Geometry check sheet. Reference: the model listing, model coordinates, mm. A direction names the side the tool comes from. Give positions to 0.01 mm unless a question says otherwise; leave off trailing zeros. Loops run counter-clockwise (first coordinate to the right, second up) from the corner with the lowest first, then second, coordinate; pieces in that order, holes last. Notation, with made-up numbers: (-25.75, -23) -> (21.25, -23) arc R20 ccw to (21.25, -14) -> close; hole circle Ø6 at (28, -33). An arc over 180 degrees is marked (long way). Answer as a JSON object with one key per item and string values.
Autodesk Inventor part; units mm, degrees
ref_plane "YZ Plane" through (0, 0, 0) normal (1, 0, 0) x (0, 1, 0)
ref_plane "XZ Plane" through (0, 0, 0) normal (0, 1, 0) x (-1, 0, 0)
ref_plane "XY Plane" through (0, 0, 0) normal (0, 0, 1) x (1, 0, 0)
sketch "Sketch1" plane through (0, 0, 0) normal (0, 0, 1) x (1, 0, 0)
  circle A0 centre (0, 0) radius 10.16
  circle A1 centre (0, 0) radius 8.7376
  dimension "d0" = 20.32
  dimension "d6" = 17.4752
extrude "Extrusion1" add sketch "Sketch1" along normal blind 12.7 contours A0 | A1
sketch "Sketch2" plane through (0, 0, 12.7) normal (0, 0, 1) x (1, 0, 0)
  circle A0 centre (0, 0) radius 10.16
  circle A1 centre (0, 0) radius 13.335 construction
  line L0 (0, 13.335) -> (15.875, 13.335)
  line L1 (15.875, 13.335) -> (15.875, -13.335)
  line L2 (15.875, -13.335) -> (0, -13.335)
  arc A2 (0, 13.335) -> (0, -13.335) centre (0, 0) ccw
  point P0 (15.875, 0)
  dimension "d3" = 3.175
  dimension "d14" = 15.875
extrude "Extrusion2" add sketch "Sketch2" along normal blind 6.35 contours A0 | L0 L1 L2 A2
sketch "Sketch4" plane through (0, 0, 19.05) normal (0, 0, 1) x (1, 0, 0)
  arc A0 (0, 13.335) -> (0, -13.335) centre (0, 0) ccw
hole "Hole2" at (0, 0, 19.05) direction (0, 0, -1) diameter 6.5278 end through all
sketch "Sketch5" plane through (0, 0, 19.05) normal (0, 0, 1) x (1, 0, 0)
  line L0 (15.875, 13.335) -> (0, 13.335)
  line L1 (0, -13.335) -> (15.875, -13.335)
  line L2 (15.875, 13.335) -> (9.525, 13.335)
  line L3 (9.525, 13.335) -> (9.525, -13.335)
  line L4 (9.525, -13.335) -> (15.875, -13.335)
  line L5 (15.875, -13.335) -> (15.875, 13.335)
  line L6 (9.525, -13.335) -> (15.875, -13.335)
  line L7 (15.875, -13.335) -> (15.875, -26.035)
  line L8 (15.875, -26.035) -> (9.525, -26.035)
  line L9 (9.525, -26.035) -> (9.525, -13.335)
  point P0 (0, 0)
  point P1 (15.875, -19.685)
  point P2 (15.875, 0)
  dimension "d22" = 6.35
  dimension "d36" = 12.7
extrude "Extrusion3" add sketch "Sketch5" along normal blind 25.4
fillet "Fillet1" radius 3.175 4 edges at (9.525, 0, 19.05) (12.7, -26.035, 19.05) (12.7, -26.035, 44.45) (12.7, 13.335, 44.45)
sketch "Sketch6" plane through (15.875, -13.335, 12.7) normal (1, 0, 0) x (0, 0, -1)
  line L0 (-25.0698, 13.335) -> (-25.0698, 0.635) construction
  line L1 (0, 26.67) -> (-28.575, 26.67) construction
  line L2 (-31.75, -9.525) -> (-31.75, 23.495)
  point P0 (12.7, 13.335)
  point P1 (-25.0698, 6.985)
  dimension "d26" = 12.7
  dimension "d35" = 13.335
  dimension "d37" = 6.6802
hole "Hole3" at (15.875, 0, 37.7698) at (15.875, -12.7, 37.7698) direction (-1, 0, 0) diameter 6.7 end through all
properties part number "EL2-020" material "ABS Plastic"
1) Tool access check on faces 4 (the face through (13, -18, 19.05)), 5 (the face through (11, 0, 12.7)), 6 (the face through (8.62, 0.187, 20.005)). Record the directions out of +Z, -Z, +X, -X, +Y, -Y that give a thin tool (end or side, any length) a straight path to the whole face; none if there is none.
Geometry check:
{"face 4": "-Z, +X, -X, -Y", "face 5": "-Z", "face 6": "+Z, -X, +Y, -Y"}
2) Draft check along X on faces 1 (the face through (15.875, -6, 28)), 2 (the face through (-4, 0, 19.05)), 3 (the face through (3.186, 0.708, 9.392)). Enter one of: pulls with the +X half, pulls with the -X half, needs draft (parallel to the pull), parting line crosses it, or undercut.
Geometry check:
{"face 1": "pulls with the +X half", "face 2": "needs draft", "face 3": "undercut"}
3) Section check B-B on z = 38. Record the cut outline in (x, y) (3 decimals), plus the area to 3 significant figures.
Geometry check:
{"outline": "(9.525, -26.035) -> (15.875, -26.035) -> (15.875, -16.042) -> (9.525, -16.042) -> close; (9.525, -9.358) -> (15.875, -9.358) -> (15.875, -3.342) -> (9.525, -3.342) -> close; (9.525, 3.342) -> (15.875, 3.342) -> (15.875, 13.335) -> (9.525, 13.335) -> close", "area": "165 mm2"}
4) Section check A-A on y = 0. Record the cut outline in (x, z) (3 decimals).
Geometry check:
{"outline": "(-13.335, 12.7) -> (-10.16, 12.7) -> (-10.16, 0) -> (-3.264, 0) -> (-3.264, 19.05) -> (-13.335, 19.05) -> close; (3.264, 0) -> (10.16, 0) -> (10.16, 12.7) -> (15.875, 12.7) -> (15.875, 34.42) -> (9.525, 34.42) -> (9.525, 22.225) arc R3.175 cw to (6.35, 19.05) -> (3.264, 19.05) -> close; (9.525, 41.12) -> (15.875, 41.12) -> (15.875, 44.45) -> (9.525, 44.45) -> close"}
5) Depth check by flat-ended pin: P1, Ø3, axis at x = -0.5, z = 13.5, coming from the -Y side (3 decimals); P2, Ø6, axis at y = 0, z = 37.77, coming from the -X side; P3, Ø7.5, axis at x = 6.5, z = 18.5, coming from the -Y side; P4, Ø10.5, axis at y = -12.7, z = 37.77, coming from the +X side (3 decimals). Enter the tip coordinate at first touch or a pass-through.
Geometry check:
{"P1": "stops at y = -13.335", "P2": "passes through", "P3": "stops at y = -25.65", "P4": "stops at x = 15.875"}
6) Section check D-D on x = -8.5. Record the cut outline in (y, z).
Geometry check:
{"outline": "(-10.27, 12.7) -> (-5.57, 12.7) -> (-5.57, 0) -> (5.57, 0) -> (5.57, 12.7) -> (10.27, 12.7) -> (10.27, 19.05) -> (-10.27, 19.05) -> close"}
7) Section check C-C on y = -12.7. Record the cut outline in (x, z) (3 decimals), plus the area to 3 significant figures.
Geometry check:
{"outline": "(-4.066, 12.7) -> (15.875, 12.7) -> (15.875, 34.42) -> (9.525, 34.42) -> (9.525, 22.225) arc R3.175 cw to (6.35, 19.05) -> (-4.066, 19.05) -> close; (9.525, 41.12) -> (15.875, 41.12) -> (15.875, 44.45) -> (9.525, 44.45) -> close", "area": "248 mm2"}
8) Material ranges on line 1 along X through (y, z) = (0, 13) (3 decimals); line 2 along Y through (x, z) = (0, 13.5) (3 decimals); line 3 along Z through (x, y) = (12.5, -12.7), recorded low to high. Write a range as from..to.
Geometry check:
{"line 1": "x = -13.335..-3.264, 3.264..15.875", "line 2": "y = -13.335..-3.264, 3.264..13.335", "line 3": "z = 12.7..34.42, 41.12..44.45"}
